The listing builds one solid part. Answer for the finished solid, in the listing's coordinates (mm). Round coordinates to 2 decimals unless told otherwise and drop trailing zeros. Loops run counter-clockwise (first coordinate to the right, second up) from the corner with the lowest first, then second, coordinate; pieces in that order, holes last. Notation, with made-up numbers: (-2.75, 52) -> (53.25, 52) arc R24 cw to (53.25, 81) -> close; hole circle Ø9 at (-29.75, 55). An arc over 180 degrees is marked (long way). Answer in a Markdown table with one row per item. Add a question column.
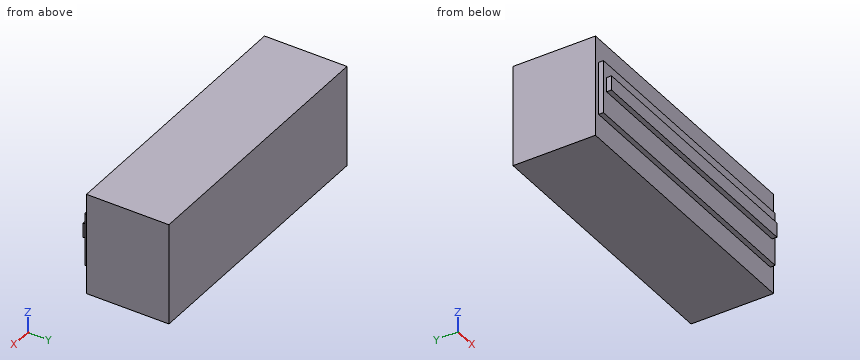
```python
from build123d import *

# Parameters (mm, degrees)
CROQUIS1_W              = 57.000000029
CROQUIS1_H              = 20.999999717
SALIENTE_EXTRUIR1_DEPTH = 16.999999993
CROQUIS2_W              = 55.000001564
CROQUIS2_H              = 11.000000872
SALIENTE_EXTRUIR2_DEPTH = 1.000000164
CROQUIS3_W              = 52.999999375
CROQUIS3_H              = 3.000000492
SALIENTE_EXTRUIR3_DEPTH = 0.999999233


with BuildPart() as part:
    # Croquis1 → Saliente-Extruir1 (new body)
    with BuildSketch(Plane(origin=(0, 9.999999776, 0), x_dir=(1, 0, 0), z_dir=(0, 1, 0))):
        with Locations((17.500000075, -10.499999859)):
            Rectangle(CROQUIS1_W, CROQUIS1_H)
    extrude(amount=-SALIENTE_EXTRUIR1_DEPTH)

    # Croquis2 → Saliente-Extruir2 (add)
    with BuildSketch(Plane.XZ.offset(7.000000216)):
        with Locations((17.500001006, 10.500000324)):
            Rectangle(CROQUIS2_W, CROQUIS2_H)
    extrude(amount=SALIENTE_EXTRUIR2_DEPTH)

    # Croquis3 → Saliente-Extruir3 (add)
    with BuildSketch(Plane.XZ.offset(8.00000038)):
        with Locations((17.500000075, 11.500000022)):
            Rectangle(CROQUIS3_W, CROQUIS3_H)
    extrude(amount=SALIENTE_EXTRUIR3_DEPTH)


solid = part.part
```
Item 1: Section B-B, the plane z = 8.25 is taken. Write down the section's boundary in (x, y).
Item 2: Flat-ended cylindrical pins translate along their axes: P1, Ø0.5, axis at x = 19, y = -7.5, coming from the +Z side; P2, Ø1.1, axis at y = -8.5, z = 11, coming from the +X side; P3, Ø0.5, axis at y = -8.5, z = 12, coming from the -X side. Find the tip coordinate at first contact, or state that the pin passes through.
Item 3: Section C-C, the plane z = 4 is taken. Write down the section's boundary in (x, y), and give its area (3 significant figures).
Item 4: Section A-A, the plane x = -5 is taken. Write down the section's boundary in (y, z), and give its area (3 significant figures).
Item 5: Consider L1, parallel to Y at x = 38, z = 1.5; L2, parallel to Y at x = 14.5, z = 5.25. Determine where each line is inside the solid, lowest interval first. Write a range as from..to.
Here are the results:
| question | item | result |
|---|---|---|
| 1 | outline | (-11, -7) -> (-10, -7) -> (-10, -8) -> (45, -8) -> (45, -7) -> (46, -7) -> (46, 10) -> (-11, 10) -> close |
| 2 | P1 | stops at z = 16 |
| 2 | P2 | stops at x = 45 |
| 2 | P3 | stops at x = -9 |
| 3 | outline | (-11, -7) -> (46, -7) -> (46, 10) -> (-11, 10) -> close |
| 3 | area | 969 mm² |
| 4 | outline | (-9, 10) -> (-8, 10) -> (-8, 5) -> (-7, 5) -> (-7, 0) -> (10, 0) -> (10, 21) -> (-7, 21) -> (-7, 16) -> (-8, 16) -> (-8, 13) -> (-9, 13) -> close |
| 4 | area | 371 mm² |
| 5 | L1 | y = -7..10 |
| 5 | L2 | y = -8..10 |
